Read the model definition and answer for the solid it produces. Units are mm, in the model's axes. A direction names the side the tool comes from. Round coordinates to 2 decimals unless told otherwise and drop trailing zeros. Write each loop counter-clockwise with the first axis right and the second up, starting at its lowest first coordinate (ties: lowest second). Pieces come first, ordered by that corner, then holes.
from build123d import *

# Parameters (mm, degrees)
SKETCH1_R           = 3.048
SKETCH1_R_2         = 3.175
BOSS_EXTRUDE1_DEPTH = 2.54
FILLET1_R           = 7.62
SKETCH2_R           = 1.4224
CUT_EXTRUDE1_DEPTH  = 160.50957323


with BuildPart() as part:
    # Sketch1 → Boss-Extrude1 (new body)
    with BuildSketch(Plane.XY):
        with BuildLine():
            Line((-19.05, 111.155403269), (-12.7, 21.997045256))
            ThreePointArc((-12.7, 21.997045256), (-17.960512242, 17.960512242), (-21.997045256, 12.7))
            Line((-21.997045256, 12.7), (-111.155403269, 19.05))
            ThreePointArc((-111.155403269, 19.05), (-112.776, 0), (-111.155403269, -19.05))
            Line((-111.155403269, -19.05), (-21.997045256, -12.7))
            ThreePointArc((-21.997045256, -12.7), (-17.960512242, -17.960512242), (-12.7, -21.997045256))
            Line((-12.7, -21.997045256), (-19.05, -111.155403269))
            ThreePointArc((-19.05, -111.155403269), (0, -112.776), (19.05, -111.155403269))
            Line((19.05, -111.155403269), (12.7, -21.997045256))
            ThreePointArc((12.7, -21.997045256), (17.960512242, -17.960512242), (21.997045256, -12.7))
            Line((21.997045256, -12.7), (111.155403269, -19.05))
            ThreePointArc((111.155403269, -19.05), (112.776, 0), (111.155403269, 19.05))
            Line((111.155403269, 19.05), (21.997045256, 12.7))
            ThreePointArc((21.997045256, 12.7), (17.960512242, 17.960512242), (12.7, 21.997045256))
            Line((12.7, 21.997045256), (19.05, 111.155403269))
            ThreePointArc((19.05, 111.155403269), (0, 112.776), (-19.05, 111.155403269))
        make_face()
        Circle(SKETCH1_R, mode=Mode.SUBTRACT)
        with Locations((9.525, 104.341147205)):
            Circle(SKETCH1_R_2, mode=Mode.SUBTRACT)
        with Locations((-9.525, 104.341147205)):
            Circle(SKETCH1_R_2, mode=Mode.SUBTRACT)
        with Locations((104.341147205, 9.525)):
            Circle(SKETCH1_R_2, mode=Mode.SUBTRACT)
        with Locations((104.341147205, -9.525)):
            Circle(SKETCH1_R_2, mode=Mode.SUBTRACT)
        with Locations((9.525, -104.341147205)):
            Circle(SKETCH1_R_2, mode=Mode.SUBTRACT)
        with Locations((-9.525, -104.341147205)):
            Circle(SKETCH1_R_2, mode=Mode.SUBTRACT)
        with Locations((-104.341147205, -9.525)):
            Circle(SKETCH1_R_2, mode=Mode.SUBTRACT)
        with Locations((-104.341147205, 9.525)):
            Circle(SKETCH1_R_2, mode=Mode.SUBTRACT)
    extrude(amount=BOSS_EXTRUDE1_DEPTH)

    # Fillet1
    fillet1_edges = [part.edges().sort_by_distance(p)[0] for p in [
        (12.7, 21.997045256, 1.27),
        (21.997045256, 12.7, 1.27),
        (21.997045256, -12.7, 1.27),
        (12.7, -21.997045256, 1.27),
        (-12.7, -21.997045256, 1.27),
        (-21.997045256, -12.7, 1.27),
        (-21.997045256, 12.7, 1.27),
        (-12.7, 21.997045256, 1.27),
    ]]
    fillet(fillet1_edges, radius=FILLET1_R)

    # Sketch2 → Cut-Extrude1 (cut, through all)
    with BuildSketch(Plane.XY):
        with Locations((0, 9.525)):
            Circle(SKETCH2_R)
        with Locations((8.248891971, 4.7625)):
            Circle(SKETCH2_R)
        with Locations((8.248891971, -4.7625)):
            Circle(SKETCH2_R)
        with Locations((0, -9.525)):
            Circle(SKETCH2_R)
        with Locations((-8.248891971, -4.7625)):
            Circle(SKETCH2_R)
        with Locations((-8.248891971, 4.7625)):
            Circle(SKETCH2_R)
    extrude(amount=CUT_EXTRUDE1_DEPTH, mode=Mode.SUBTRACT)


solid = part.part
Q1. Which of the six approach directions +Z, -Z, +X, -X, +Y, -Y give full straight-line access (tool end or side, diameter ignored) to faces 5 (the flat face through (68.154, -15.987, 1.252)), 6 (the flat face through (-68.154, 15.987, 1.252)), 7 (the cylindrical face through (-107.513, -9.385, 1.252)), 8 (the flat face through (-15.987, -68.154, 1.252)), 9 (the flat face through (16.07, -69.34, 1.25))?
Verdict:
face 5: +Z, -Z, -Y
face 6: +Z, -Z, +Y
face 7: +Z, -Z
face 8: +Z, -Z, -X
face 9: +Z, -Z, +X
Q2. Section A-A (y = 0) is taken. Determine the outline of the cut face in (x, z), then the cut area to 3 significant figures.
Verdict:
outline: (-112.78, 0) - (-3.05, 0) - (-3.05, 2.54) - (-112.78, 2.54) - close; (3.05, 0) - (112.78, 0) - (112.78, 2.54) - (3.05, 2.54) - close
area: 557 mm2
Q3. Section B-B (z = 0.5) is taken. State how many separate pieces and enclosed holes the cut face has, then the cut area to 3 significant figures.
Verdict:
separate pieces: 1
enclosed holes: 15
area: 13,000 mm2
Q4. Flat-ended cylindrical pins translate along their axes: pin 1 Ø1 at (x, z) = (1, 1) entering from +Y; pin 2 Ø1 at (x, z) = (-20.5, 1.5) entering from +Y. Find the tip coordinate at first contact, or state that the pin passes through.
Verdict:
pin 1: stops at y = 112.77
pin 2: stops at y = 15.67
Q5. Determine the mould class of faces 1 (the flat face through (-69.34, -16.07, 1.25)), 2 (the cylindrical face through (-10.21, -107.44, 1.25)), 3 (the flat face through (69.34, 16.07, 1.25)), 4 (the flat face through (-1, -8, 2.54)) for opening direction Y: pulls with the +Y half, pulls with the -Y half, needs draft (parallel to the pull), parting line crosses it, or undercut.
Verdict:
face 1: pulls with the -Y half
face 2: undercut
face 3: pulls with the +Y half
face 4: needs draft
Q6. Section C-C (x = -69) is taken. Determine the outline of the cut face in (y, z), then the cut area to 3 significant figures.
Verdict:
outline: (-16.05, 0) - (16.05, 0) - (16.05, 2.54) - (-16.05, 2.54) - close
area: 81.5 mm2
Q7. Section D-D (y = 53) is taken. Determine the outline of the cut face in (x, z), then the cut area to 3 significant figures.
Verdict:
outline: (-14.91, 0) - (14.91, 0) - (14.91, 2.54) - (-14.91, 2.54) - close
area: 75.7 mm2
Q8. Straight lines are drawn through the part: probe 1 along Y at (x, z) = (0, 0.65); probe 2 along Y at (x, z) = (0.5, 2.1); probe 3 along X at (y, z) = (4, 1.65). For each, find the intervals that lie inside material, in ascending order.
Verdict:
probe 1: y = -112.78 to -10.95, -8.1 to -3.05, 3.05 to 8.1, 10.95 to 112.78
probe 2: y = -112.77 to -10.86, -8.19 to -3.01, 3.01 to 8.19, 10.86 to 112.77
probe 3: x = -112.71 to -9.45, -7.05 to 7.05, 9.45 to 112.71
